Autodesk Fusion 360 part; units mm, degrees
sketch "Sketch1" plane through (0, 0, 0) normal (0, 0, 1) x (1, 0, 0)
  line L0 (-32.5, 32.5) -> (32.5, 32.5)
  line L1 (32.5, 32.5) -> (32.5, -32.5)
  line L2 (32.5, -32.5) -> (-32.5, -32.5)
  line L3 (-32.5, -32.5) -> (-32.5, 32.5)
  point P0 (-18, 24)
  point P1 (18, 24)
  point P2 (18, -24)
  point P3 (-18, -24)
  dimension "d1" = 65
  dimension "d2" = 65
  dimension "d3" = 32.5
  dimension "d4" = 32.5
  dimension "d5" = 14.5
  dimension "d6" = 14.5
  dimension "d7" = 14.5
  dimension "d8" = 14.5
  dimension "d9" = 8.5
  dimension "d10" = 8.5
  dimension "d11" = 8.5
  dimension "d12" = 8.5
extrude "Extrude1" add sketch "Sketch1" along normal blind 5
hole "Hole1" at (-18, -24, 0) at (18, -24, 0) at (18, 24, 0) at (-18, 24, 0) direction (0, 0, 1) diameter 3.5 depth 5 tip angle 180 countersink diameter 6 countersink angle 90
sketch "Sketch2" plane through (0, 32.5, 0) normal (0, 1, 0) x (-1, 0, 0)
  line L0 (-32.5, 0) -> (32.5, 0)
  line L1 (32.5, 0) -> (32.5, 5)
  line L2 (32.5, 5) -> (-32.5, 5)
  line L3 (-32.5, 5) -> (-32.5, 0)
  line L4 (-25.5, 5) -> (24.5, 5)
  line L5 (24.5, 5) -> (24.5, 0)
  line L6 (24.5, 0) -> (-25.5, 0)
  line L7 (-25.5, 0) -> (-25.5, 5)
  dimension "d20" = 50
  dimension "d21" = 7
extrude "Extrude2" add sketch "Sketch2" along normal blind 85 contours L0 L2 L4 L5 L6 L7
sketch "Sketch3" plane through (0, 0, 5) normal (0, 0, 1) x (-1, 0, 0)
  circle A0 centre (-18, -24) radius 1.75
  circle A1 centre (18, 24) radius 1.75
  circle A2 centre (-18, 24) radius 1.75
  circle A3 centre (18, -24) radius 1.75
  line L0 (32.5, 32.5) -> (-32.5, 32.5)
  line L1 (-32.5, 32.5) -> (-32.5, -32.5)
  line L2 (-32.5, -32.5) -> (-25.5, -32.5)
  line L3 (-25.5, -32.5) -> (-25.5, -117.5)
  line L4 (-25.5, -117.5) -> (24.5, -117.5)
  line L5 (24.5, -117.5) -> (24.5, -32.5)
  line L6 (24.5, -32.5) -> (32.5, -32.5)
  line L7 (32.5, -32.5) -> (32.5, 32.5)
  line L8 (24.5, -32.5) -> (-25.5, -32.5) construction
  line L9 (2.5, -112.5) -> (-3.5, -112.5)
  line L10 (2.5, -93.5) -> (-3.5, -93.5)
  arc A4 (-3.5, -93.5) -> (-3.5, -112.5) centre (-3.5, -103) ccw
  arc A5 (2.5, -112.5) -> (2.5, -93.5) centre (2.5, -103) ccw
  circle A6 centre (19.5, -37.5) radius 1.75
  circle A7 centre (-20.5, -37.5) radius 1.75
  circle A8 centre (-20.5, -112.5) radius 1.75
  circle A9 centre (19.5, -112.5) radius 1.75
  point P0 (12, -103)
  point P1 (-13, -103)
  dimension "d27" = 19
  dimension "d29" = 22
  dimension "d30" = 3.5
  dimension "d31" = 3.5
  dimension "d32" = 3.5
  dimension "d33" = 3.5
  dimension "d34" = 5
  dimension "d35" = 5
  dimension "d36" = 5
  dimension "d37" = 5
  dimension "d39" = 5
  dimension "d40" = 5
  dimension "d48" = 22
  dimension "d49" = 5
extrude "Extrude3" cut sketch "Sketch3" against normal blind 5 contours L9 L10 A4 A5 | A6 | A7 | A8 | A9
fillet "Fillet1" radius 4 4 edges at (25.5, 32.5, 2.5) (25.5, 117.5, 2.5) (-24.5, 117.5, 2.5) (-24.5, 32.5, 2.5)
fillet "Fillet2" radius 4 4 edges at (32.5, -32.5, 2.5) (-32.5, -32.5, 2.5) (-32.5, 32.5, 2.5) (32.5, 32.5, 2.5)
equation "d3 = ( 65 / 2 ) * 1 mm"
equation "d4 = ( 65 / 2 ) * 1 mm"
equation "d5 = 13 mm + ( 3 / 2 ) * 1 mm"
equation "d9 = 7 mm + ( ( 3 / 2 ) * 1 mm )"
equation "d21 = ( ( 64 - 50 ) / 2 ) * 1 mm"
equation "d27 = 23.5 mm - 4.5 mm"
Model file for the job. Use its own axes, mm. A direction names the side the tool comes from. Coordinates: 2 decimals unless noted, no trailing zeros. Order: outer loops, then holes, each group sorted by start corner. A loop starts at its lowest first (then second) coordinate and runs counter-clockwise, first axis right, second up. Notation, with made-up numbers: (54.5, 11) - (77.5, 11) arc R23 ccw to (77.5, 27) - close; hole circle Ø3 at (-21.75, -32.5). An arc over 180 degrees is marked (long way). Return JSON: item names as keys, results as strings. Group by question number.
1) Saw through at C-C, the plane x = -9. Write the cut outline in (y, z).
2) Flat gauge pins, fed straight in: P1, Ø4, axis at x = -18, y = -24, coming from the +Z side; P2, Ø3, axis at x = 18, y = -24, coming from the -Z side. Where does each tip first touch, or does it go through?
3) Saw through at A-A, the plane y = -24. Write the cut outline in (x, z), plus the area to 3 significant figures.
4) Saw through at B-B, the plane z = 3.95. Count the separate pieces of the cut face and the enclosed holes in it, plus the area to 3 significant figures.
5) Saw through at D-D, the plane y = 102. Write the cut outline in (x, z), plus the area to 3 significant figures.
6) Tool access for faces 1 (the cylindrical face through (13, 103, 3)), 2 (the flat face through (25.5, 74, 2)), 3 (the flat face through (-32.5, 0, 2)): list every direction of +Z, -Z, +X, -X, +Y, -Y with a clear straight run to the whole face (end or side of a thin tool).
7) Probe line 1 (X direction, y = 24, z = 2.3); line 2 (Y direction, x = 18, z = 2.4); line 3 (Y direction, x = -3, z = 1.7). List the from-to ranges inside material, lowest first. Write a range as from..to.
8) Mould opens along Y. For faces 4 (the flat face through (0, 27, 5)), 5 (the conical face through (-16, -24, 1)), 6 (the cylindrical face through (26.473, 33.885, 2.535)) say: released by +Y, released by -Y, zero draft, split by the parting line, or undercut.
Values found:
{
 "1": {"outline": "(-32.5, 0) - (96.07, 0) - (96.07, 5) - (-32.5, 5) - close; (109.93, 0) - (117.5, 0) - (117.5, 5) - (109.93, 5) - close"},
 "2": {"P1": "stops at z = 5", "P2": "passes through"},
 "3": {"outline": "(-32.5, 0) - (-21, 0) - (-19.75, 1.25) - (-19.75, 5) - (-32.5, 5) - close; (-16.25, 1.25) - (-15, 0) - (15, 0) - (16.25, 1.25) - (16.25, 5) - (-16.25, 5) - close; (19.75, 1.25) - (21, 0) - (32.5, 0) - (32.5, 5) - (19.75, 5) - close", "area": "287 mm²"},
 "4": {"separate pieces": "1", "enclosed holes": "9", "area": "7,990 mm²"},
 "5": {"outline": "(-24.5, 0) - (-11.95, 0) - (-11.95, 5) - (-24.5, 5) - close; (12.95, 0) - (25.5, 0) - (25.5, 5) - (12.95, 5) - close", "area": "126 mm²"},
 "6": {"face 1": "+Z, -Z", "face 2": "+Z, -Z, +X, +Y", "face 3": "+Z, -Z, -X, +Y, -Y"},
 "7": {"line 1": "x = -32.5..-19.75, -16.25..16.25, 19.75..32.5", "line 2": "y = -32.5..-25.75, -22.25..22.25, 25.75..117.5", "line 3": "y = -32.5..93.51, 112.49..117.5"},
 "8": {"face 4": "zero draft", "face 5": "undercut", "face 6": "released by +Y"}
}
